from build123d import *

# Parameters (mm, degrees)
SKIZZE1_W                        = 42
SKIZZE1_H                        = 42
SKIZZE1_R                        = 1.25
SKIZZE1_R_2                      = 11
AUFSATZ_LINEAR_AUSTRAGEN1_DEPTH  = 15
SKIZZE2_W                        = 50
SKIZZE2_H                        = 30
AUFSATZ_LINEAR_AUSTRAGEN2_DEPTH  = 50
SKIZZE3_R                        = 15
SCHNITT_LINEAR_AUSTRAGEN9_DEPTH  = 30
SKIZZE4_R                        = 17.5
SCHNITT_LINEAR_AUSTRAGEN10_DEPTH = 11.75
SKIZZE5_W                        = 50
SKIZZE5_H                        = 20
SCHNITT_LINEAR_AUSTRAGEN3_DEPTH  = 4
SKIZZE6_R                        = 2
SCHNITT_LINEAR_AUSTRAGEN4_DEPTH  = 11
SKIZZE8_R                        = 32.5
SKIZZE8_R_2                      = 26.25
SCHNITT_LINEAR_AUSTRAGEN5_DEPTH  = 4
SKIZZE10_R                       = 20
AUFSATZ_LINEAR_AUSTRAGEN3_DEPTH  = 50
SKIZZE11_R                       = 3.5
SCHNITT_LINEAR_AUSTRAGEN6_DEPTH  = 8
SKIZZE12_R                       = 10
SCHNITT_LINEAR_AUSTRAGEN7_DEPTH  = 65
SKIZZE13_R                       = 2
SCHNITT_LINEAR_AUSTRAGEN8_DEPTH  = 15


with BuildPart() as part:
    # Skizze1 → Aufsatz-Linear austragen1 (new body)
    # profile 1 of 4: a face of its own
    with BuildSketch(Plane(origin=(0, 0, 0), x_dir=(1, 0, 0), z_dir=(0, 1, 0))):
        with BuildLine():
            ThreePointArc((46, 0), (0, 46), (-46, 0))
            Line((-46, 0), (46, 0))
        make_face()
    # profile 2 of 4: a face of its own
    with BuildSketch(Plane(origin=(0, 0, 0), x_dir=(1, 0, 0), z_dir=(0, 1, 0))):
        with BuildLine():
            Line((-46, 68), (-46, 0))
            ThreePointArc((-46, 0), (0, 46), (46, 0))
            Line((46, 0), (46, 110))
            Line((46, 110), (-4, 110))
            Line((-4, 110), (-4, 68))
            Line((-4, 68), (-46, 68))
        make_face()
    # profile 3 of 4: a face of its own
    with BuildSketch(Plane(origin=(0, 0, 0), x_dir=(1, 0, 0), z_dir=(0, 1, 0))):
        with BuildLine():
            Line((46, 0), (-46, 0))
            ThreePointArc((-46, 0), (0, -46), (46, 0))
        make_face()
    # profile 4 of 4: a face of its own
    with BuildSketch(Plane(origin=(0, 0, 0), x_dir=(1, 0, 0), z_dir=(0, 1, 0))):
        with Locations((-25, 89)):
            Rectangle(SKIZZE1_W, SKIZZE1_H)
        with Locations(Location((-40.5, 73.5, 0), (0, 0, 270))):
            Circle(SKIZZE1_R, mode=Mode.SUBTRACT)
        with Locations(Location((-25, 89, 0), (0, 0, 270))):
            Circle(SKIZZE1_R_2, mode=Mode.SUBTRACT)
        with Locations(Location((-40.5, 104.5, 0), (0, 0, 270))):
            Circle(SKIZZE1_R, mode=Mode.SUBTRACT)
        with Locations(Location((-9.5, 73.5, 0), (0, 0, 270))):
            Circle(SKIZZE1_R, mode=Mode.SUBTRACT)
        with Locations(Location((-9.5, 104.5, 0), (0, 0, 270))):
            Circle(SKIZZE1_R, mode=Mode.SUBTRACT)
    extrude(amount=AUFSATZ_LINEAR_AUSTRAGEN1_DEPTH)

    # Skizze2 → Aufsatz-Linear austragen2 (add)
    with BuildSketch(Plane(origin=(0, 15, 0), x_dir=(1, 0, 0), z_dir=(0, 1, 0))):
        with Locations((21, 82.5)):
            Rectangle(SKIZZE2_W, SKIZZE2_H)
    extrude(amount=AUFSATZ_LINEAR_AUSTRAGEN2_DEPTH)

    # Skizze3 → Schnitt-Linear austragen9 (cut)
    with BuildSketch(Plane(origin=(0, 0, -97.5), x_dir=(-1, 0, 0), z_dir=(0, 0, -1))):
        with Locations((-21, 40)):
            Circle(SKIZZE3_R)
    extrude(amount=-SCHNITT_LINEAR_AUSTRAGEN9_DEPTH, mode=Mode.SUBTRACT)

    # Skizze4 → Schnitt-Linear austragen10 (cut)
    with BuildSketch(Plane(origin=(0, 0, -97.5), x_dir=(-1, 0, 0), z_dir=(0, 0, -1))):
        with Locations((-21, 40)):
            Circle(SKIZZE4_R)
    schnitt_linear_austragen10 = extrude(amount=-SCHNITT_LINEAR_AUSTRAGEN10_DEPTH, mode=Mode.SUBTRACT)

    # Skizze5 → Schnitt-Linear austragen3 (cut)
    with BuildSketch(Plane(origin=(0, 15, 0), x_dir=(1, 0, 0), z_dir=(0, 1, 0))):
        with Locations((21, 32.5)):
            Rectangle(SKIZZE5_W, SKIZZE5_H)
    extrude(amount=-SCHNITT_LINEAR_AUSTRAGEN3_DEPTH, mode=Mode.SUBTRACT)

    # Skizze6 → Schnitt-Linear austragen4 (cut)
    with BuildSketch(Plane(origin=(0, 11, 0), x_dir=(1, 0, 0), z_dir=(0, 1, 0))):
        with Locations(Location((0, 32.5, 0), (0, 0, 270))):
            Circle(SKIZZE6_R)
        with Locations(Location((42, 32.5, 0), (0, 0, 90))):
            Circle(SKIZZE6_R)
        with Locations(Location((10, 32.5, 0), (0, 0, 270))):
            Circle(SKIZZE6_R)
        with Locations(Location((32, 32.5, 0), (0, 0, 90))):
            Circle(SKIZZE6_R)
    extrude(amount=-SCHNITT_LINEAR_AUSTRAGEN4_DEPTH, mode=Mode.SUBTRACT)

    # Skizze8 → Schnitt-Linear austragen5 (cut)
    with BuildSketch(Plane.XZ):
        Circle(SKIZZE8_R)
        with Locations(Location((0, 0, 0), (0, 0, 270))):
            Circle(SKIZZE8_R_2, mode=Mode.SUBTRACT)
    extrude(amount=-SCHNITT_LINEAR_AUSTRAGEN5_DEPTH, mode=Mode.SUBTRACT)

    # Skizze10 → Aufsatz-Linear austragen3 (add)
    with BuildSketch(Plane.XZ):
        with Locations(Location((0, 0, 0), (0, 0, 270))):
            Circle(SKIZZE10_R)
    extrude(amount=AUFSATZ_LINEAR_AUSTRAGEN3_DEPTH)

    # Skizze11 → Schnitt-Linear austragen6 (cut)
    with BuildSketch(Plane.XZ):
        with Locations(Location((0, -32.5, 0), (0, 0, 3.086650162))):
            Circle(SKIZZE11_R)
        with Locations(Location((10, -32.5, 0), (0, 0, 168.965324237))):
            Circle(SKIZZE11_R)
        with Locations(Location((32, -32.5, 0), (0, 0, 270))):
            Circle(SKIZZE11_R)
        with Locations(Location((42, -32.5, 0), (0, 0, 270))):
            Circle(SKIZZE11_R)
    extrude(amount=-SCHNITT_LINEAR_AUSTRAGEN6_DEPTH, mode=Mode.SUBTRACT)

    # Skizze12 → Schnitt-Linear austragen7 (cut)
    with BuildSketch(Plane.XZ.offset(50)):
        with Locations(Location((0, 0, 0), (0, 0, 270))):
            Circle(SKIZZE12_R)
    extrude(amount=-SCHNITT_LINEAR_AUSTRAGEN7_DEPTH, mode=Mode.SUBTRACT)

    # Skizze13 → Schnitt-Linear austragen8 (cut)
    with BuildSketch(Plane.XZ.offset(50)):
        with Locations(Location((15, 0, 0), (0, 0, 270))):
            Circle(SKIZZE13_R)
        with Locations(Location((7.5, -12.990381057, 0), (0, 0, 270))):
            Circle(SKIZZE13_R)
        with Locations(Location((-7.5, -12.990381057, 0), (0, 0, 270))):
            Circle(SKIZZE13_R)
        with Locations(Location((-15, 0, 0), (0, 0, 270))):
            Circle(SKIZZE13_R)
        with Locations(Location((-7.5, 12.990381057, 0), (0, 0, 270))):
            Circle(SKIZZE13_R)
        with Locations(Location((7.5, 12.990381057, 0), (0, 0, 270))):
            Circle(SKIZZE13_R)
    extrude(amount=-SCHNITT_LINEAR_AUSTRAGEN8_DEPTH, mode=Mode.SUBTRACT)

    # Spiegeln2: Schnitt-Linear austragen10 across plane
    add(schnitt_linear_austragen10.mirror(Plane(origin=(0, 0, -82.5), x_dir=(1, 0, 0), z_dir=(0, 0, -1))), mode=Mode.SUBTRACT)


solid = part.part
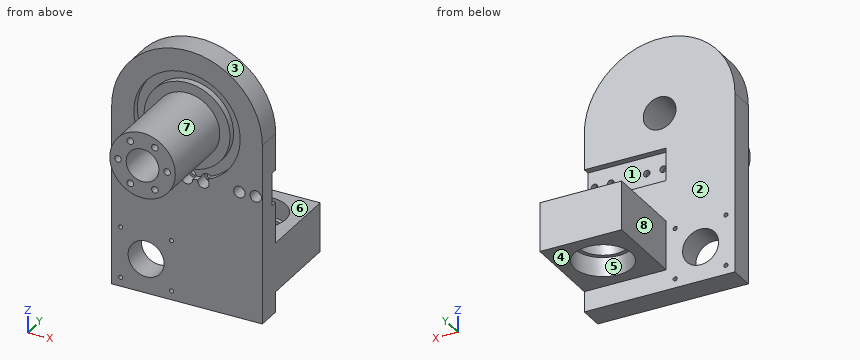
Here's how the part is built. I have some questions about the finished solid (model axes, mm). Face numbers are marked on the shaded views. A direction names the side the tool comes from. Coordinates: 2 decimals unless noted, no trailing zeros. Write each loop counter-clockwise with the first axis right and the second up, starting at its lowest first coordinate (ties: lowest second). Pieces come first, ordered by that corner, then holes.
1) If we section it at B-B (y = 42.5): List the corners of the cut face in (x, z) for me.
Filled in:
outline: (-4, -97.5) - (3.68, -97.5) - (3.68, -85.75) - (6.21, -85.75) - (6.21, -79.25) - (3.68, -79.25) - (3.68, -67.5) - (-4, -67.5) - close; (35.79, -85.75) - (38.32, -85.75) - (38.32, -97.5) - (46, -97.5) - (46, -67.5) - (38.32, -67.5) - (38.32, -79.25) - (35.79, -79.25) - close
2) I'm going to push flat-ended pins straight in: pin 1 (3 mm diameter, centred on x = 29, y = 2.5, fed in from +Z); pin 2 (3 mm diameter, centred on x = 7.5, z = 12.99, fed in from +Y); pin 3 (11 mm diameter, centred on x = 32, z = -32.5, fed in from +Y); pin 4 (3 mm diameter, centred on x = 42, z = -32.5, fed in from +Y). Where does each tip first touch, or does it pass through?
Filled in:
pin 1: stops at z = 36.87
pin 2: stops at y = 15
pin 3: stops at y = 11
pin 4: passes through
3) Which directions (+Z, -Z, +X, -X, +Y, -Y) give clear straight access to the entire face, cutting with the end or side of a thin tool? Please do the marked faces 5, 6, 7 and 8.
Filled in:
face 5: -Z
face 6: +Z, +X, -X, +Y
face 7: -Y
face 8: +Z, -Z, -X, +Y
4) If we section it at A-A (z = -89): List the corners of the cut face in (x, y) for me, plus the area to 3 significant figures.
Filled in:
outline: (-46, 0) - (-36, 0) - (-36, 15) - (-46, 15) - close; (-14, 0) - (46, 0) - (46, 65) - (-4, 65) - (-4, 15) - (-14, 15) - close; hole circle Ø35 at (21, 40)
area: 2,590 mm2
5) If we section it at D-D (y = -21.5): List the corners of the cut face in (x, z) for me, plus the area to 3 significant figures.
Filled in:
outline: circle Ø40 at (0, 0); hole circle Ø20 at (0, 0)
area: 942 mm2
6) If I drill on line 1 (X direction, y = 3, z = -32.5); line 2 (Y direction, x = 21, z = -73); line 3 (Y direction, x = 20, z = -26), over which ranges is the centre line in solid material (lowest first)?
Filled in:
line 1: x = -46 to -3.5, 3.5 to 6.5, 13.5 to 28.5, 35.5 to 38.5, 45.5 to 46
line 2: y = 0 to 22.5, 57.5 to 65
line 3: y = 0 to 11
7) Thinking about a two-plate mould opening in Z: for the marked faces 1, 2, 3 and 4, which applies, +Z half, -Z half, draft (parallel to the pull), parting line (faces both ways), or undercut?
Filled in:
face 1: undercut
face 2: draft
face 3: +Z half
face 4: -Z half
8) If we section it at C-C (z = 5.5): List the corners of the cut face in (x, y) for me, plus the area to 3 significant figures.
Filled in:
outline: (-45.67, 0) - (-32.03, 0) - (-32.03, 4) - (-25.67, 4) - (-25.67, 0) - (-19.23, 0) - (-19.23, -50) - (-8.35, -50) - (-8.35, 15) - (-45.67, 15) - close; (8.35, -50) - (19.23, -50) - (19.23, 0) - (25.67, 0) - (25.67, 4) - (32.03, 4) - (32.03, 0) - (45.67, 0) - (45.67, 15) - (8.35, 15) - close
area: 2,160 mm2
